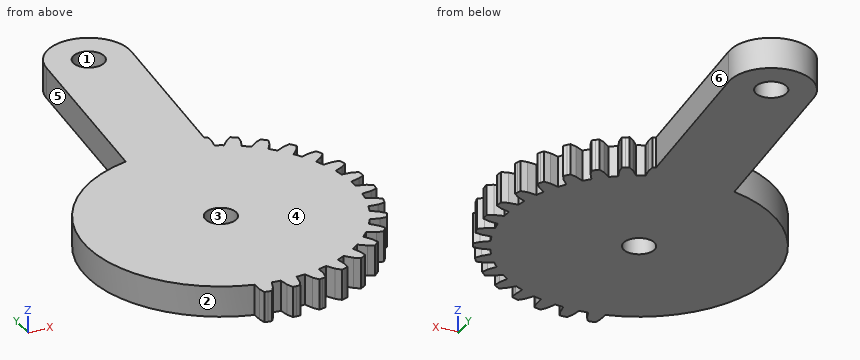
from build123d import *

# Parameters (mm, degrees)
BOSS_EXTRUDE1_DEPTH = 3
SKETCH2_R           = 1.5
CUT_EXTRUDE1_DEPTH  = 7
BOSS_EXTRUDE4_START = -3
SKETCH4_R           = 1.5
BOSS_EXTRUDE4_DEPTH = 3


with BuildPart() as part:
    # Sketch1 → Boss-Extrude1 (new body)
    with BuildSketch(Plane.XY):
        with BuildLine():
            Line((-0.612376666, 13.878994029), (-0.776800125, 12.976770845))
            ThreePointArc((-0.776800125, 12.976770845), (-12.944544292, 1.199488673), (-3.148049012, -12.613080013))
            Line((-3.148049012, -12.613080013), (-3.15220825, -13.530153864))
            Line((-3.15220825, -13.530153864), (-3.012443123, -14.183623882))
            Line((-3.012443123, -14.183623882), (-2.664368008, -14.253109945))
            Line((-2.664368008, -14.253109945), (-2.314696368, -14.314055356))
            Line((-2.314696368, -14.314055356), (-1.948308671, -13.755201698))
            Line((-1.948308671, -13.755201698), (-1.620901759, -12.89855331))
            ThreePointArc((-1.620901759, -12.89855331), (-1.199488673, -12.944544292), (-0.776800125, -12.976770845))
            Line((-0.776800125, -12.976770845), (-0.612376666, -13.878994029))
            Line((-0.612376666, -13.878994029), (-0.354916505, -14.495655703))
            Line((-0.354916505, -14.495655703), (0, -14.5))
            Line((0, -14.5), (0.354916505, -14.495655703))
            Line((0.354916505, -14.495655703), (0.612376666, -13.878994029))
            Line((0.612376666, -13.878994029), (0.776800125, -12.976770845))
            ThreePointArc((0.776800125, -12.976770845), (1.199488673, -12.944544292), (1.620901759, -12.89855331))
            Line((1.620901759, -12.89855331), (1.948308671, -13.755201698))
            Line((1.948308671, -13.755201698), (2.314696368, -14.314055356))
            Line((2.314696368, -14.314055356), (2.664368008, -14.253109945))
            Line((2.664368008, -14.253109945), (3.012443123, -14.183623882))
            Line((3.012443123, -14.183623882), (3.15220825, -13.530153864))
            Line((3.15220825, -13.530153864), (3.148049012, -12.613080013))
            ThreePointArc((3.148049012, -12.613080013), (3.557618871, -12.503733361), (3.963405777, -12.381091012))
            Line((3.963405777, -12.381091012), (4.442646693, -13.162992471))
            Line((4.442646693, -13.162992471), (4.905485034, -13.64500702))
            Line((4.905485034, -13.64500702), (5.23800416, -13.520847326))
            Line((5.23800416, -13.520847326), (5.567384604, -13.388585761))
            Line((5.567384604, -13.388585761), (5.584695163, -12.720560537))
            Line((5.584695163, -12.720560537), (5.412094866, -11.819865869))
            ThreePointArc((5.412094866, -11.819865869), (5.794598625, -11.637122788), (6.170940766, -11.442005509))
            Line((6.170940766, -11.442005509), (6.78569571, -12.122533323))
            Line((6.78569571, -12.122533323), (7.32922329, -12.511294336))
            Line((7.32922329, -12.511294336), (7.633266362, -12.328148468))
            Line((7.633266362, -12.328148468), (7.932735479, -12.137615409))
            Line((7.932735479, -12.137615409), (7.82700198, -11.477783777))
            Line((7.82700198, -11.477783777), (7.491838321, -10.624140369))
            ThreePointArc((7.491838321, -10.624140369), (7.834250273, -10.374223955), (8.168331768, -10.113276232))
            Line((8.168331768, -10.113276232), (8.897665999, -10.669255841))
            Line((8.897665999, -10.669255841), (9.503373637, -10.951524529))
            Line((9.503373637, -10.951524529), (9.768586833, -10.7156293))
            Line((9.768586833, -10.7156293), (10.027946562, -10.473313122))
            Line((10.027946562, -10.473313122), (9.802769632, -9.844144857))
            Line((9.802769632, -9.844144857), (9.316456206, -9.066622511))
            ThreePointArc((9.316456206, -9.066622511), (9.607115924, -8.758043367), (9.887560028, -8.440151462))
            Line((9.887560028, -8.440151462), (10.706636943, -8.852649649))
            Line((10.706636943, -8.852649649), (11.353897993, -9.01881369))
            Line((11.353897993, -9.01881369), (11.571249796, -8.738202227))
            Line((11.571249796, -8.738202227), (11.781667951, -8.452354718))
            Line((11.781667951, -8.452354718), (11.444715722, -7.875275391))
            Line((11.444715722, -7.875275391), (10.82381335, -7.200351698))
            ThreePointArc((10.82381335, -7.200351698), (11.052822764, -6.843618117), (11.27007929, -6.479607457))
            Line((11.27007929, -6.479607457), (12.151006207, -6.73457709))
            Line((12.151006207, -6.73457709), (12.81777897, -6.778977966))
            Line((12.81777897, -6.778977966), (12.979867725, -6.463206159))
            Line((12.979867725, -6.463206159), (13.134178769, -6.143561512))
            Line((13.134178769, -6.143561512), (12.696925744, -5.638222867))
            Line((12.696925744, -5.638222867), (11.962578511, -5.088881543))
            ThreePointArc((11.962578511, -5.088881543), (12.122138982, -4.69614166), (12.268809519, -4.298408191))
            Line((12.268809519, -4.298408191), (13.181587529, -4.387166586))
            Line((13.181587529, -4.387166586), (13.845165858, -4.308292279))
            Line((13.845165858, -4.308292279), (13.946471826, -3.968113356))
            Line((13.946471826, -3.968113356), (14.039420882, -3.625556687))
            Line((14.039420882, -3.625556687), (13.516757188, -3.209167425))
            Line((13.516757188, -3.209167425), (12.693972409, -2.804115631))
            ThreePointArc((12.693972409, -2.804115631), (12.778650296, -2.388743732), (12.849740155, -1.97083179))
            Line((12.849740155, -1.97083179), (13.763285697, -1.890356385))
            Line((13.763285697, -1.890356385), (14.401072228, -1.690892865))
            Line((14.401072228, -1.690892865), (14.438145556, -1.337891212))
            Line((14.438145556, -1.337891212), (14.466567355, -0.984087877))
            Line((14.466567355, -0.984087877), (13.876291677, -0.670827635))
            Line((13.876291677, -0.670827635), (12.993088302, -0.423858924))
            ThreePointArc((12.993088302, -0.423858924), (13, 0), (12.993088302, 0.423858924))
            Line((12.993088302, 0.423858924), (13.876291677, 0.670827635))
            Line((13.876291677, 0.670827635), (14.466567355, 0.984087877))
            Line((14.466567355, 0.984087877), (14.438145556, 1.337891212))
            Line((14.438145556, 1.337891212), (14.401072228, 1.690892865))
            Line((14.401072228, 1.690892865), (13.763285697, 1.890356385))
            Line((13.763285697, 1.890356385), (12.849740155, 1.97083179))
            ThreePointArc((12.849740155, 1.97083179), (12.778650296, 2.388743732), (12.693972409, 2.804115631))
            Line((12.693972409, 2.804115631), (13.516757188, 3.209167425))
            Line((13.516757188, 3.209167425), (14.039420882, 3.625556687))
            Line((14.039420882, 3.625556687), (13.946471826, 3.968113356))
            Line((13.946471826, 3.968113356), (13.845165858, 4.308292279))
            Line((13.845165858, 4.308292279), (13.181587529, 4.387166586))
            Line((13.181587529, 4.387166586), (12.268809519, 4.298408191))
            ThreePointArc((12.268809519, 4.298408191), (12.122138982, 4.69614166), (11.962578511, 5.088881543))
            Line((11.962578511, 5.088881543), (12.696925744, 5.638222867))
            Line((12.696925744, 5.638222867), (13.134178769, 6.143561512))
            Line((13.134178769, 6.143561512), (12.979867725, 6.463206159))
            Line((12.979867725, 6.463206159), (12.81777897, 6.778977966))
            Line((12.81777897, 6.778977966), (12.151006207, 6.73457709))
            Line((12.151006207, 6.73457709), (11.27007929, 6.479607457))
            ThreePointArc((11.27007929, 6.479607457), (11.052822764, 6.843618117), (10.82381335, 7.200351698))
            Line((10.82381335, 7.200351698), (11.444715722, 7.875275391))
            Line((11.444715722, 7.875275391), (11.781667951, 8.452354718))
            Line((11.781667951, 8.452354718), (11.571249796, 8.738202228))
            Line((11.571249796, 8.738202228), (11.353897993, 9.01881369))
            Line((11.353897993, 9.01881369), (10.706636943, 8.852649649))
            Line((10.706636943, 8.852649649), (9.887560028, 8.440151462))
            ThreePointArc((9.887560028, 8.440151462), (9.607115924, 8.758043367), (9.316456206, 9.066622511))
            Line((9.316456206, 9.066622511), (9.802769632, 9.844144857))
            Line((9.802769632, 9.844144857), (10.027946562, 10.473313122))
            Line((10.027946562, 10.473313122), (9.768586833, 10.7156293))
            Line((9.768586833, 10.7156293), (9.503373637, 10.951524529))
            Line((9.503373637, 10.951524529), (8.897665999, 10.669255841))
            Line((8.897665999, 10.669255841), (8.168331768, 10.113276232))
            ThreePointArc((8.168331768, 10.113276232), (7.834250273, 10.374223955), (7.491838321, 10.624140369))
            Line((7.491838321, 10.624140369), (7.82700198, 11.477783777))
            Line((7.82700198, 11.477783777), (7.932735479, 12.137615409))
            Line((7.932735479, 12.137615409), (7.633266362, 12.328148468))
            Line((7.633266362, 12.328148468), (7.32922329, 12.511294336))
            Line((7.32922329, 12.511294336), (6.78569571, 12.122533323))
            Line((6.78569571, 12.122533323), (6.170940766, 11.442005509))
            ThreePointArc((6.170940766, 11.442005509), (5.794598625, 11.637122788), (5.412094866, 11.819865869))
            Line((5.412094866, 11.819865869), (5.584695163, 12.720560537))
            Line((5.584695163, 12.720560537), (5.567384604, 13.388585761))
            Line((5.567384604, 13.388585761), (5.23800416, 13.520847326))
            Line((5.23800416, 13.520847326), (4.905485034, 13.64500702))
            Line((4.905485034, 13.64500702), (4.442646693, 13.162992471))
            Line((4.442646693, 13.162992471), (3.963405777, 12.381091012))
            ThreePointArc((3.963405777, 12.381091012), (3.557618871, 12.503733361), (3.148049012, 12.613080013))
            Line((3.148049012, 12.613080013), (3.15220825, 13.530153864))
            Line((3.15220825, 13.530153864), (3.012443123, 14.183623882))
            Line((3.012443123, 14.183623882), (2.664368008, 14.253109945))
            Line((2.664368008, 14.253109945), (2.314696368, 14.314055356))
            Line((2.314696368, 14.314055356), (1.948308671, 13.755201698))
            Line((1.948308671, 13.755201698), (1.620901759, 12.89855331))
            ThreePointArc((1.620901759, 12.89855331), (1.199488673, 12.944544292), (0.776800125, 12.976770845))
            Line((0.776800125, 12.976770845), (0.612376666, 13.878994029))
            Line((0.612376666, 13.878994029), (0.354916505, 14.495655703))
            Line((0.354916505, 14.495655703), (0, 14.5))
            Line((0, 14.5), (-0.354916505, 14.495655703))
            Line((-0.354916505, 14.495655703), (-0.612376666, 13.878994029))
        make_face()
    extrude(amount=BOSS_EXTRUDE1_DEPTH)

    # Sketch2 → Cut-Extrude1 (cut)
    with BuildSketch(Plane.XY.offset(3)):
        Circle(SKETCH2_R)
    extrude(amount=-CUT_EXTRUDE1_DEPTH, mode=Mode.SUBTRACT)

    # Sketch4 → Boss-Extrude4 (add)
    with BuildSketch(Plane.XY.offset(3).offset(BOSS_EXTRUDE4_START)):
        with BuildLine():
            Line((-1.122617562, 31.236832903), (-2.841640129, 12.68562499))
            ThreePointArc((-2.841640129, 12.68562499), (-1.815067202, 12.872666043), (-0.776800125, 12.976770845))
            Line((-0.776800125, 12.976770845), (-0.612376666, 13.878994029))
            Line((-0.612376666, 13.878994029), (-0.354916505, 14.495655703))
            Line((-0.354916505, 14.495655703), (0, 14.5))
            Line((0, 14.5), (0.354916505, 14.495655703))
            Line((0.354916505, 14.495655703), (0.612376666, 13.878994029))
            Line((0.612376666, 13.878994029), (0.776800125, 12.976770845))
            ThreePointArc((0.776800125, 12.976770845), (1.199488673, 12.944544292), (1.620901759, 12.89855331))
            Line((1.620901759, 12.89855331), (1.948308671, 13.755201698))
            Line((1.948308671, 13.755201698), (2.314696368, 14.314055356))
            Line((2.314696368, 14.314055356), (2.664368008, 14.253109945))
            Line((2.664368008, 14.253109945), (3.012443123, 14.183623882))
            Line((3.012443123, 14.183623882), (3.15220825, 13.530153864))
            Line((3.15220825, 13.530153864), (3.148049012, 12.613080013))
            ThreePointArc((3.148049012, 12.613080013), (3.557618871, 12.503733361), (3.963405777, 12.381091012))
            Line((3.963405777, 12.381091012), (4.442646693, 13.162992471))
            Line((4.442646693, 13.162992471), (4.905485034, 13.64500702))
            Line((4.905485034, 13.64500702), (5.23800416, 13.520847326))
            Line((5.23800416, 13.520847326), (5.268878609, 13.508449799))
            Line((5.268878609, 13.508449799), (6.843255849, 30.498686027))
            ThreePointArc((6.843255849, 30.498686027), (3.229392581, 34.85069617), (-1.122617562, 31.236832903))
        make_face()
        with Locations((2.860319143, 30.867759465)):
            Circle(SKETCH4_R, mode=Mode.SUBTRACT)
    extrude(amount=BOSS_EXTRUDE4_DEPTH)


solid = part.part
Geometry: final body of the model. Coordinates: model frame, mm. Face numbers are marked on the shaded views. A direction names the side the tool comes from. Round coordinates to 2 decimals unless told otherwise and drop trailing zeros. Loops run counter-clockwise (first coordinate to the right, second up) from the corner with the lowest first, then second, coordinate; pieces in that order, holes last. Notation, with made-up numbers: (0, 54) - (20, 54) arc R22 ccw to (20, 84) - close; hole circle Ø7 at (59.25, 67.25). An arc over 180 degrees is marked (long way). Write each question's results on one line, items separated by ' | '. Start each with the question number.
1) Cut plane B-B on y = 24. Return loops of the section in (x, z), then the cut area to 3 significant figures.
2) Line query: probe 1 along X at (y, z) = (-8.5, 1.2); probe 2 along Y at (x, z) = (0, 1.15); probe 3 along X at (y, z) = (23, 1.55). Output: solid intervals per line, ascending. Write a range as [from, to].
3) Cut plane A-A on z = 1.55. Count the separate pieces of the cut face and the enclosed holes in it, then the cut area to 3 significant figures.
4) Access query for the marked faces 5 and 6. Directions: +Z, -Z, +X, -X, +Y, -Y. A direction counts if a zero-diameter tool reaches every point of the face in a straight line with its end or side. Return the directions, or none.
5) Mould query, pull axis Y, two halves, no side actions, for the marked faces 1, 2, 3 and 4. Classes: released by +Y, released by -Y, zero draft, split by the parting line, or undercut.
6) First-contact query: P1, Ø1.5, axis at y = 23, z = 2.5, coming from the -X side; P2, Ø1.5, axis at y = 20.5, z = 1.5, coming from the -X side; P3, Ø2.5, axis at x = 2.86, y = 30.87, coming from the -Z side. Flat tips, straight axial feed; report the tip coordinate or a pass-through.
7) Cut plane C-C on x = -4. Return loops of the section in (y, z).
Verdict:
1) outline: (-1.79, 0) - (6.24, 0) - (6.24, 3) - (-1.79, 3) - close | area: 24.1 mm2
2) probe 1: x = [-9.84, 9.84], [10.01, 11.75] | probe 2: y = [-14.5, -1.5], [1.5, 33.66] | probe 3: x = [-1.89, 6.15]
3) separate pieces: 1 | enclosed holes: 2 | area: 717 mm2
4) face 5: +Z, -Z, -X, +Y | face 6: +Z, -Z, +X
5) face 1: undercut | face 2: split by the parting line | face 3: undercut | face 4: zero draft
6) P1: stops at x = -1.96 | P2: stops at x = -2.19 | P3: passes through
7) outline: (-12.37, 0) - (12.37, 0) - (12.37, 3) - (-12.37, 3) - close
